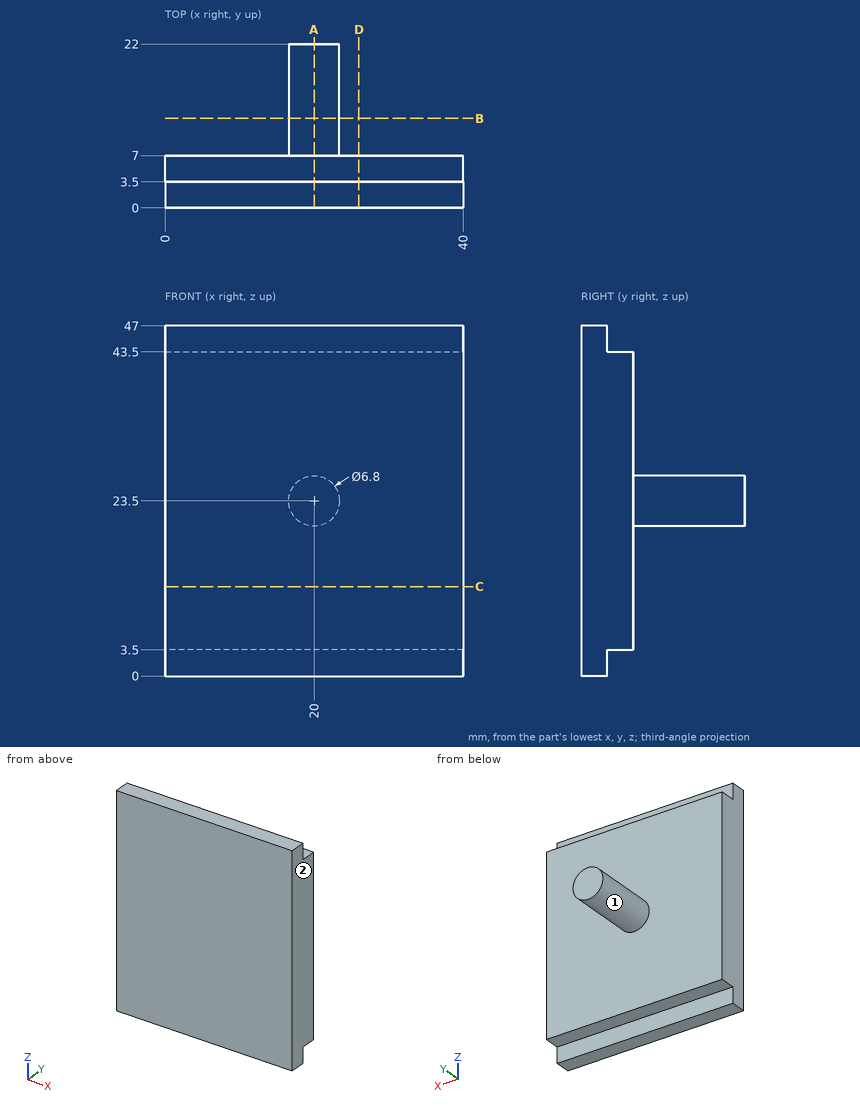
Geometry check sheet. Reference: drawing and pictorial views, mm from the part's lowest x, y, z. A direction names the side the tool comes from. Round coordinates to 2 decimals unless told otherwise and drop trailing zeros. Order: outer loops, then holes, each group sorted by start corner. A loop starts at its lowest first (then second) coordinate and runs counter-clockwise, first axis right, second up. Notation, with made-up numbers: M 29,-28.5 L 64,-28.5 A19 cw 64,-8.5 Z; hole C 42,3 d8. An arc over 180 degrees is marked long. Answer as CSV lines item,"result".
1) Sectioned sample at D-D on x = 26. Record the cut outline in (y, z), and give its area (4 significant figures).
Entries:
outline,"M 0,0 L 3.5,0 L 3.5,3.5 L 7,3.5 L 7,43.5 L 3.5,43.5 L 3.5,47 L 0,47 Z"
area,"304.5 mm2"
2) Sectioned sample at A-A on x = 20. Record the cut outline in (y, z), and give its area (4 significant figures).
Entries:
outline,"M 0,0 L 3.5,0 L 3.5,3.5 L 7,3.5 L 7,20.1 L 22,20.1 L 22,26.9 L 7,26.9 L 7,43.5 L 3.5,43.5 L 3.5,47 L 0,47 Z"
area,"406.5 mm2"
3) Sectioned sample at B-B on y = 12. Record the cut outline in (x, z), and give its area (3 significant figures).
Entries:
outline,"C 20,23.5 d6.8"
area,"36.3 mm2"
4) Tool access check on the marked faces 1 and 2. Record the directions out of +Z, -Z, +X, -X, +Y, -Y that give a thin tool (end or side, any length) a straight path to the whole face; none if there is none.
Entries:
face 1,"+Y"
face 2,"+Z, -Z, +X, +Y, -Y"
5) Thickness scan on probe 1 along Y at (x, z) = (8, 5); probe 2 along Z at (x, y) = (30, 4.5); probe 3 along Y at (x, z) = (9, 44.5). Record the ranges inside material, lowest first. Write a range as [from, to].
Entries:
probe 1,"[0, 7]"
probe 2,"[3.5, 43.5]"
probe 3,"[0, 3.5]"
6) Gauge pin test, flat ends, axial feed: pin 1 Ø1 at (x, y) = (22.5, 4.5) entering from -Z; pin 2 Ø2 at (x, z) = (18, 29.5) entering from +Y; pin 3 Ø2 at (y, z) = (14.5, 25.5) entering from -X. Record the tip position at first contact, or that the pin passes through.
Entries:
pin 1,"z = 3.5"
pin 2,"y = 7"
pin 3,"x = 16.75"
7) Sectioned sample at C-C on z = 12. Record the cut outline in (x, y), and give its area (3 significant figures).
Entries:
outline,"M 0,0 L 40,0 L 40,7 L 0,7 Z"
area,"280 mm2"
